from build123d import *

# Parameters (mm, degrees)
SKETCH_R           = 150
PAD_DEPTH          = 10
SKETCH001_R        = 6
POCKET_DEPTH       = 858.764807
POLARPATTERN_COUNT = 4
SKETCH002_R        = 32.5
POCKET001_DEPTH    = 10.001


with BuildPart() as part:
    # Sketch → Pad (new body)
    with BuildSketch(Plane.XY):
        Circle(SKETCH_R)
    extrude(amount=PAD_DEPTH)

    # Sketch001 (on Face3 of Pad) → Pocket (cut, through all)
    with BuildSketch(Plane.XY.offset(10)):
        with Locations((0, 50)):
            Circle(SKETCH001_R)
    pocket = extrude(amount=-POCKET_DEPTH, mode=Mode.SUBTRACT)

    # PolarPattern: Pocket ×4 about axis
    polarpattern_axis = Axis((0, 0, 10), (0, 0, 1))
    for i in range(1, POLARPATTERN_COUNT):
        add(pocket.rotate(polarpattern_axis, i * 360 / POLARPATTERN_COUNT), mode=Mode.SUBTRACT)

    # Sketch002 (on Face3 of PolarPattern) → Pocket001 (cut, through all)
    with BuildSketch(Plane.XY.offset(10)):
        Circle(SKETCH002_R)
    extrude(amount=-POCKET001_DEPTH, mode=Mode.SUBTRACT)


solid = part.part
Part model, mm, in its own coordinate system. Round coordinates to 2 decimals unless told otherwise and drop trailing zeros. Write each loop counter-clockwise with the first axis right and the second up, starting at its lowest first coordinate (ties: lowest second). Pieces come first, ordered by that corner, then holes. Notation, with made-up numbers: M 50,-27.5 L 66,-27.5 A33 cw 66,0.5 Z; hole C 48,24 d4. An arc over 180 degrees is marked long. Return JSON: item names as keys, results as strings. Group by question number.
(1) Saw through at A-A on y = 0. Write the cut outline in (x, z).
(2) Two-plate mould, pull along Y, no slides. Class faces 1 (the face through (-1.301, 44.143, 5.07)), 2 (the face through (-2, 35, 10)), 3 (the face through (-19.527, 148.724, 4.93)), 4 (the face through (31, 9.76, 5.07)): +Y half, -Y half, draft (parallel to the pull), parting line (faces both ways), or undercut.
(3) Pin check, flat tips, straight feed: pin 1 Ø3 at (y, z) = (-66, 3.5) entering from -X; pin 2 Ø11 at (x, y) = (50, 0) entering from -Z; pin 3 Ø2 at (x, z) = (37.5, 4) entering from -Y; pin 4 Ø3 at (x, z) = (62.5, 5.5) entering from -Y. Stop position of each tip, or through.
(4) Drill centre lines: probe 1 along Y at (x, z) = (0, 2); probe 2 along Y at (x, z) = (-50, 4.75). Where is each one in solid material? Low to high.
(5) Saw through at C-C on z = 2.75. Write the cut outline in (x, y), then the cut area to 3 significant figures.
(6) Saw through at D-D on y = -50. Write the cut outline in (x, z), then the cut area to 3 significant figures.
Returned:
{
 "1": {"outline": "M -150,0 L -56,0 L -56,10 L -150,10 Z; M -44,0 L -32.5,0 L -32.5,10 L -44,10 Z; M 32.5,0 L 44,0 L 44,10 L 32.5,10 Z; M 56,0 L 150,0 L 150,10 L 56,10 Z"},
 "2": {"face 1": "undercut", "face 2": "draft", "face 3": "parting line", "face 4": "undercut"},
 "3": {"pin 1": "x = -135.42", "pin 2": "through", "pin 3": "y = -145.49", "pin 4": "y = -137.04"},
 "4": {"probe 1": "-150 to -56, -44 to -32.5, 32.5 to 44, 56 to 150", "probe 2": "-141.42 to -6, 6 to 141.42"},
 "5": {"outline": "C 0,0 d300; hole C -50,0 d12; hole C 0,0 d65; hole C 0,-50 d12; hole C 0,50 d12; hole C 50,0 d12", "area": "66,900 mm²"},
 "6": {"outline": "M -141.42,0 L -6,0 L -6,10 L -141.42,10 Z; M 6,0 L 141.42,0 L 141.42,10 L 6,10 Z", "area": "2,710 mm²"}
}
